Input: part model. Units: mm. Frame: model coordinates. A direction names the side the tool comes from. Coordinates: 2 decimals unless noted, no trailing zeros. Write each loop counter-clockwise with the first axis right and the second up, starting at its lowest first coordinate (ties: lowest second). Pieces come first, ordered by that corner, then holes. Notation, with made-up numbers: (-12, 52.25) -> (1, 52.25) arc R22 ccw to (1, 78.25) -> close; hole circle Ø5 at (45.25, 39.25). An arc over 180 degrees is marked (long way). One line per question, with ' | ' between items. Start each with the question number.
```python
from build123d import *

# Parameters (mm, degrees)
SKETCH1_R           = 5.5
SKETCH1_R_2         = 1.5
BOSS_EXTRUDE1_DEPTH = 2
SKETCH2_W           = 0.4
SKETCH2_H           = 4.013393125
CUT_EXTRUDE1_DEPTH  = 3
CHAMFER1_SIZE       = 0.8
LPATTERN1_COUNT     = 4
LPATTERN1_PITCH     = 12
SKETCH3_W           = 2.911545786
SKETCH3_H           = 2.4
BOSS_EXTRUDE2_DEPTH = 0.8


with BuildPart() as part:
    # Sketch1 → Boss-Extrude1 (new body)
    with BuildSketch(Plane.XY):
        Circle(SKETCH1_R)
        Circle(SKETCH1_R_2, mode=Mode.SUBTRACT)
    extrude(amount=BOSS_EXTRUDE1_DEPTH)

    # Sketch2 → Cut-Extrude1 (cut, through all)
    with BuildSketch(Plane.XY.offset(2)):
        with Locations((0, 3.493303437)):
            Rectangle(SKETCH2_W, SKETCH2_H)
    extrude(amount=-CUT_EXTRUDE1_DEPTH, mode=Mode.SUBTRACT)

    # Chamfer1
    chamfer1_edges = [part.edges().sort_by_distance(p)[0] for p in [
        (-3.817721834, -3.959166579, 2),
        (-3.817721834, -3.959166579, 0),
    ]]
    chamfer(chamfer1_edges, length=CHAMFER1_SIZE)


with BuildPart() as lpattern1_1:
    # LPattern1: pattern copy
    add(part.part.moved(Location(Vector(1, 0, 0) * (1 * LPATTERN1_PITCH))))


with BuildPart() as lpattern1_2:
    # LPattern1: pattern copy
    add(part.part.moved(Location(Vector(1, 0, 0) * (2 * LPATTERN1_PITCH))))


with BuildPart() as lpattern1_3:
    # LPattern1: pattern copy
    add(part.part.moved(Location(Vector(1, 0, 0) * (3 * LPATTERN1_PITCH))))


with BuildPart() as part_1:
    add(part.part)

    add(lpattern1_1.part)  # Boss-Extrude2 merges LPattern1_1

    add(lpattern1_2.part)  # Boss-Extrude2 merges LPattern1_2

    add(lpattern1_3.part)  # Boss-Extrude2 merges LPattern1_3
    # Sketch3 → Boss-Extrude2 (add)
    with BuildSketch(Plane(origin=(0, 0, 0), x_dir=(-1, 0, 0), z_dir=(0, 0, -1))):
        with Locations((-18, 0)):
            Rectangle(SKETCH3_W, SKETCH3_H)
        with Locations((-6, 0)):
            Rectangle(SKETCH3_W, SKETCH3_H)
        with Locations((-30, 0)):
            Rectangle(SKETCH3_W, SKETCH3_H)
    extrude(amount=-BOSS_EXTRUDE2_DEPTH)


solid = part_1.part
```
1) Ray query, line 1 (X direction, y = -3.25, z = 0.9); line 2 (X direction, y = -2, z = 0.8); line 3 (Y direction, x = 24, z = 1). Return the intervals inside material, ascending.
2) First-contact query: P1, Ø1.4, axis at x = 6, y = -0.5, coming from the +Z side; P2, Ø1.5, axis at x = 36, y = 0, coming from the +Z side; P3, Ø1, axis at y = 3, z = 1, coming from the +X side; P4, Ø0.6, axis at y = 3, z = 1, coming from the +X side. Flat tips, straight axial feed; report the tip coordinate or a pass-through.
3) Section A-A, the plane z = 0.45. Return loops of the section in (x, y), then the cut area to 3 significant figures.
4) Pull-direction query (X, two-part tool) for faces 1 (the face through (36, -2, 2)), 2 (the face through (32.89, 3.81, 0.22)); classes: released by +X, released by -X, zero draft, split by the parting line, or undercut.
5) Access query for faces 3 (the face through (35.94, -1.5, 0.99)), 4 (the face through (24.2, 3, 1)), 5 (the face through (20.89, 3.81, 0.22)). Directions: +Z, -Z, +X, -X, +Y, -Y. A direction counts if a zero-diameter tool reaches every point of the face in a straight line with its end or side. Return the directions, or none.
Answer block:
1) line 1: x = -4.44 to 4.44, 7.56 to 16.44, 19.56 to 28.44, 31.56 to 40.44 | line 2: x = -5.12 to 5.12, 6.88 to 17.12, 18.88 to 29.12, 30.88 to 41.12 | line 3: y = -5.5 to -1.5
2) P1: stops at z = 1.38 | P2: passes through | P3: stops at x = 40.9 | P4: stops at x = 40.79
3) outline: (-0.2, 1.49) -> (-0.2, 5.15) arc R5.15 ccw (long way) to (5.01, -1.2) -> (6.99, -1.2) arc R5.15 ccw to (17.01, -1.2) -> (18.99, -1.2) arc R5.15 ccw to (29.01, -1.2) -> (30.99, -1.2) arc R5.15 ccw (long way) to (36.2, 5.15) -> (36.2, 1.49) arc R1.5 cw (long way) to (35.8, 1.49) -> (35.8, 5.15) arc R5.15 ccw to (30.99, 1.2) -> (29.01, 1.2) arc R5.15 ccw to (24.2, 5.15) -> (24.2, 1.49) arc R1.5 cw (long way) to (23.8, 1.49) -> (23.8, 5.15) arc R5.15 ccw to (18.99, 1.2) -> (17.01, 1.2) arc R5.15 ccw to (12.2, 5.15) -> (12.2, 1.49) arc R1.5 cw (long way) to (11.8, 1.49) -> (11.8, 5.15) arc R5.15 ccw to (6.99, 1.2) -> (5.01, 1.2) arc R5.15 ccw to (0.2, 5.15) -> (0.2, 1.49) arc R1.5 cw (long way) to start | area: 312 mm2
4) face 1: zero draft | face 2: undercut
5) face 3: +Z, -Z | face 4: +Z, -Z, +Y | face 5: -Z, +Y
